Autodesk Inventor part; units mm, degrees
ref_plane "Work Plane1" through (0, 8.5, 0) normal (0, 1, 0) x (1, 0, 0)
ref_plane "YZ Plane" through (0, 0, 0) normal (1, 0, 0) x (0, 1, 0)
ref_plane "XZ Plane" through (0, 0, 0) normal (0, 1, 0) x (-1, 0, 0)
sketch "Sketch1" plane through (0, 0, 0) normal (0, 1, 0) x (-1, 0, 0)
  circle A0 centre (0, 0) radius 5
  dimension "Diameter" = 10
extrude "Extrusion1" add sketch "Sketch1" along normal mid plane 7
fillet "Fillet1" radius 2 1 edges at (5, 3.5, 0)
sketch "Sketch2" plane through (0, -3.5, 0) normal (0, -1, 0) x (1, 0, 0)
  circle A0 centre (0, 0) radius 1.5
  dimension "d4" = 3
extrude "Extrusion2" cut sketch "Sketch2" against normal through all
sketch "Sketch3" plane through (0, 0, 0) normal (0, 0, 1) x (1, 0, 0)
  circle A0 centre (0, -1) radius 1.25
  line L0 (-5, -3.5) -> (5, -3.5)
  point P0 (0, 0)
  dimension "d7" = 2.5
  dimension "d8" = 2.5
extrude "Extrusion3" cut sketch "Sketch3" along normal blind 7
ref_plane "Work Plane1" through (0, 8.5, 0) normal (0, 1, 0) x (1, 0, 0)
sketch "Sketch4" plane through (0, 8.5, 0) normal (0, 1, 0) x (1, 0, 0)
  circle A0 centre (3.5, 0) radius 0.25
  point P0 (0, 0)
  dimension "d12" = 0.5
  dimension "d13" = 3.5
extrude "Extrusion4" cut sketch "Sketch4" against normal blind 9
thread "Thread1"
properties part number "Lower Lock Cap" material "Mild Steel S355 J2"
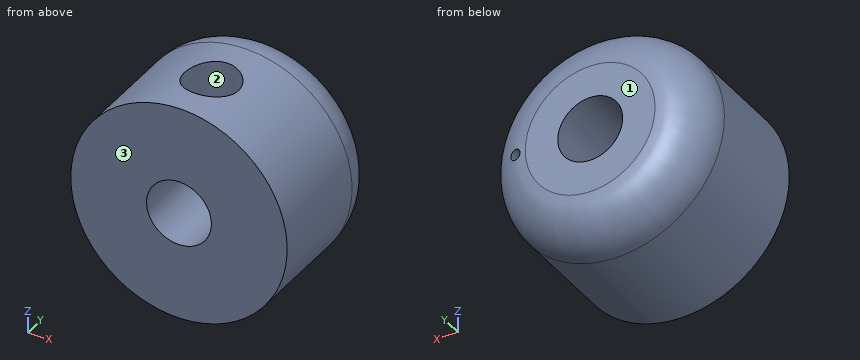
Could you check a few things on this model? Use its own coordinates, in mm. Face numbers are marked on the shaded views. Give positions to 0.01 mm unless a question says otherwise; leave off trailing zeros. Order: outer loops, then holes, each group sorted by start corner. A loop starts at its lowest first (then second) coordinate and runs counter-clockwise, first axis right, second up. Notation, with made-up numbers: (13, 52) -> (39, 52) arc R24 cw to (39, 78) -> close; hole circle Ø8 at (40, 32). An arc over 180 degrees is marked (long way). Return JSON: item names as keys, results as strings.
1. Imagine slicing it at C-C on y = 0.5. List the corners of the cut face in (x, z) for me, then the cut area to 3 significant figures.
Answer list:
{"outline": "circle Ø10 at (0, 0); hole circle Ø3 at (0, 0); hole circle Ø0.5 at (3.5, 0)", "area": "71.3 mm2"}
2. Thinking about a two-plate mould opening in Y: for the marked faces 1, 2 and 3, which applies, pulls with the +Y half, pulls with the -Y half, needs draft (parallel to the pull), parting line crosses it, or undercut?
Answer list:
{"face 1": "pulls with the +Y half", "face 2": "undercut", "face 3": "pulls with the -Y half"}
3. I need wall thicknesses on line 1 (Y direction, x = 0, z = 1.75); line 2 (Z direction, x = 0, y = 0.5); line 3 (Y direction, x = -0.5, z = 2.25). Which ranges of each line are inside material? Lowest first, please. Write a range as from..to.
Answer list:
{"line 1": "y = -3.5..-2.25, 0.25..3.5", "line 2": "z = -5..-1.5, 1.5..5", "line 3": "y = -3.5..-2.15, 0.15..3.5"}
4. Imagine slicing it at B-B on y = -0.25. List the corners of the cut face in (x, z) for me, then the cut area to 3 significant figures.
Answer list:
{"outline": "(-1, 1.12) -> (-1, 4.9) arc R5 ccw (long way) to (1, 4.9) -> (1, 1.12) arc R1.5 cw (long way) to start; hole circle Ø0.5 at (3.5, 0)", "area": "64.1 mm2"}
5. For pin 1 Ø2 at (y, z) = (-0.5, -3) entering from -X; pin 2 Ø2 at (x, y) = (0, -1) entering from +Z, each with a flat end and sliding along its axis, tell me the tip position at first contact or that it passes through.
Answer list:
{"pin 1": "stops at x = -4.58", "pin 2": "stops at z = -1.12"}
6. Imagine slicing it at D-D on y = 2.25. List the corners of the cut face in (x, z) for me, then the cut area to 3 significant figures.
Answer list:
{"outline": "circle Ø9.71 at (0, 0); hole circle Ø3 at (0, 0); hole circle Ø0.5 at (3.5, 0)", "area": "66.8 mm2"}
7. Imagine slicing it at A-A on x = 0. List the corners of the cut face in (y, z) for me, then the cut area to 3 significant figures.
Answer list:
{"outline": "(-3.5, -5) -> (1.5, -5) arc R2 ccw to (3.5, -3) -> (3.5, -1.5) -> (-3.5, -1.5) -> close; (-3.5, 1.5) -> (-2.25, 1.5) -> (-2.25, 5) -> (-3.5, 5) -> close; (0.25, 1.5) -> (3.5, 1.5) -> (3.5, 3) arc R2 ccw to (1.5, 5) -> (0.25, 5) -> close", "area": "38.5 mm2"}
